Verification items for the finished model (mm, model axes). A direction names the side the tool comes from. Coordinates: 2 decimals unless noted, no trailing zeros. Order: outer loops, then holes, each group sorted by start corner. A loop starts at its lowest first (then second) coordinate and runs counter-clockwise, first axis right, second up. Notation, with made-up numbers: M -40,84 L -23,84 A27 ccw -23,119 Z; hole C -35,-1.75 d6. An arc over 180 degrees is marked long. Return JSON: item names as keys, results as strings. Group by question number.
Q1. Go/stop test with a flat-tipped pin: pin 1 Ø1.5 at (x, y) = (36.5, -4) entering from -Z. Record where the tip stops, or that it passes through.
Q2. Section check A-A, the plane x = -25. Enter the section's corners in (y, z), then the cut area to 3 significant figures.
Q3. Mould release check, pull along Y, two halves, no side actions. Record for faces 1 (the face through (-36, 4.25, 1)), 2 (the face through (-59.248, -8.037, 1.521)), 3 (the face through (-60, 1, 1)): pulls with the +Y half, pulls with the -Y half, needs draft (parallel to the pull), parting line crosses it, or undercut.
Q4. Thickness scan on probe 1 along X at (y, z) = (8.25, 1.05); probe 2 along Y at (x, z) = (-10.5, 1.5); probe 3 along X at (y, z) = (0.75, 0.75). Record the ranges inside material, lowest first.
Q5. Section check B-B, the plane x = 31.5. Enter the section's corners in (y, z).
Q6. Access from +Z, -Z, +X, -X, +Y, -Y to the whole of each face (thin tool, end or side, straight path). Record for faces 4 (the face through (-1, 0, 3)), 5 (the face through (42.3, 5, 1)), 6 (the face through (-39, 1.75, 1)).
Q7. Section check C-C, the plane z = 0.8. Count the separate pieces of the cut face and the enclosed holes in it, then the cut area to 3 significant figures.
from build123d import *

# Parameters (mm, degrees)
SKETCH1_R           = 1.1
SKETCH1_R_2         = 1.6
SKETCH1_R_3         = 1.375
BOSS_EXTRUDE1_DEPTH = 3
FILLET1_R           = 2.5


with BuildPart() as part:
    # Sketch1 → Boss-Extrude1 (new body)
    with BuildSketch(Plane.XY):
        Polygon((-60, -8.75), (60, -8.75), (60, 8.75), (39.8, 8.75), (39.8, 6.25), (42.3, 6.25), (42.3, 4.25), (39.8, 4.25), (39.8, 1.75), (37.6, 1.75), (37.6, 4.25), (35.1, 4.25), (35.1, 6.25), (37.6, 6.25), (37.6, 8.75), (-37.6, 8.75), (-37.6, 6.25), (-35.1, 6.25), (-35.1, 4.25), (-37.6, 4.25), (-37.6, 1.75), (-39.8, 1.75), (-39.8, 4.25), (-42.3, 4.25), (-42.3, 6.25), (-39.8, 6.25), (-39.8, 8.75), (-60, 8.75), align=None)
        with Locations((-10.5, 6.25)):
            Circle(SKETCH1_R, mode=Mode.SUBTRACT)
        with Locations((-10.5, -6.25)):
            Circle(SKETCH1_R, mode=Mode.SUBTRACT)
        with Locations((10.5, -6.25)):
            Circle(SKETCH1_R, mode=Mode.SUBTRACT)
        with Locations((10.5, 6.25)):
            Circle(SKETCH1_R, mode=Mode.SUBTRACT)
        with Locations((-31.5, 6.25)):
            Circle(SKETCH1_R, mode=Mode.SUBTRACT)
        with Locations((-31.5, -6.25)):
            Circle(SKETCH1_R, mode=Mode.SUBTRACT)
        with Locations((31.5, -6.25)):
            Circle(SKETCH1_R, mode=Mode.SUBTRACT)
        with Locations((31.5, 6.25)):
            Circle(SKETCH1_R, mode=Mode.SUBTRACT)
        with Locations((25, 2)):
            Circle(SKETCH1_R_2, mode=Mode.SUBTRACT)
        with Locations((-25, 2)):
            Circle(SKETCH1_R_2, mode=Mode.SUBTRACT)
        with Locations((22.5, -2.5)):
            Circle(SKETCH1_R_2, mode=Mode.SUBTRACT)
        with Locations((-22.5, -2.5)):
            Circle(SKETCH1_R_3, mode=Mode.SUBTRACT)
    extrude(amount=BOSS_EXTRUDE1_DEPTH)

    # Fillet1
    fillet1_edges = [part.edges().sort_by_distance(p)[0] for p in [
        (60, -8.75, 1.5),
        (-60, -8.75, 1.5),
    ]]
    fillet(fillet1_edges, radius=FILLET1_R)


solid = part.part
Numbers:
{
 "1": {"pin 1": "stops at z = 0"},
 "2": {"outline": "M -8.75,0 L 0.4,0 L 0.4,3 L -8.75,3 Z; M 3.6,0 L 8.75,0 L 8.75,3 L 3.6,3 Z", "area": "42.9 mm2"},
 "3": {"face 1": "undercut", "face 2": "pulls with the -Y half", "face 3": "needs draft"},
 "4": {"probe 1": "x = -60 to -39.8, -37.6 to 37.6, 39.8 to 60", "probe 2": "y = -8.75 to -7.35, -5.15 to 5.15, 7.35 to 8.75", "probe 3": "x = -60 to -26, -24 to 24, 26 to 60"},
 "5": {"outline": "M -8.75,0 L -7.35,0 L -7.35,3 L -8.75,3 Z; M -5.15,0 L 5.15,0 L 5.15,3 L -5.15,3 Z; M 7.35,0 L 8.75,0 L 8.75,3 L 7.35,3 Z"},
 "6": {"face 4": "+Z, +X, -X, +Y, -Y", "face 5": "+Z, -Z", "face 6": "+Z, -Z, +Y"},
 "7": {"separate pieces": "1", "enclosed holes": "12", "area": "1,990 mm2"}
}
